Part model, mm, in its own coordinate system. A direction names the side the tool comes from. Give positions to 0.01 mm unless a question says otherwise; leave off trailing zeros. Write each loop counter-clockwise with the first axis right and the second up, starting at its lowest first coordinate (ties: lowest second). Pieces come first, ordered by that corner, then holes. Notation, with made-up numbers: M 28.25,-5 L 75.25,-5 A8 cw 75.25,10 Z; hole C 1,68 d8. An arc over 180 degrees is marked long. Answer as CSV lines item,"result". Start each with the question number.
Item 1: 3-axis set-ups, long thin cutter, end or side, ignore diameter. For faces 4 (the flat face through (-7, 1, 3.5)), 5 (the flat face through (0, 0, 16)), 6 (the flat face through (6, 1, 23.5)): which of +Z, -Z, +X, -X, +Y, -Y reach the whole face in a straight line?
Item 2: Band-saw the part on D-D, the plane y = -27. List the corners of the cut face in (x, z).
Item 3: Two-plate mould, pull along Z, no slides. Class faces 1 (the flat face through (0, 3, 16)), 2 (the cylindrical face through (0.301, -6.898, 45.386)), 3 (the flat face through (-5, 1, 6)): +Z half, -Z half, draft (parallel to the pull), parting line (faces both ways), or undercut.
Item 4: Pin check, flat tips, straight feed: pin 1 (1.5 mm diameter, centred on x = 7, y = 1, fed in from +Z); pin 2 (1.5 mm diameter, centred on x = 4.5, y = -30.5, fed in from -Z); pin 3 (1 mm diameter, centred on x = 3, y = -14, fed in from -Z). Stop position of each tip, or through.
Item 5: Wall check: L1, parallel to Y at x = 20.4, z = 10; L2, parallel to Y at x = 2.5, z = 4; L3, parallel to Y at x = 13, z = 38.5. Give the ranges that are in metal, low to high. Write a range as from..to.
Item 6: Band-saw the part on C-C, the plane y = -22. List the corners of the cut face in (x, z).
Item 7: Band-saw the part on B-B, the plane z = 26. List the corners of the cut face in (x, y).
Item 8: Band-saw the part on A-A, the plane x = -10.5. List the corners of the cut face in (y, z).
from build123d import *

# Parameters (mm, degrees)
SKETCH_2_W               = 43
SKETCH_2_H               = 32
EXTRUDE_1_DEPTH          = 3
EXTRUDE_2_DEPTH          = 43
SKETCH_4_W               = 3
SKETCH_4_H               = 5
CUT_EXTRUDE_1_DEPTH      = 67.543791262
SKETCH_5_R               = 0.4
CUT_EXTRUDE_2_DEPTH      = 3
CUT_EXTRUDE_START        = -40
SKETCH_5_3_R             = 0.4
CUT_EXTRUDE_3_DEPTH      = 3
CUT_EXTRUDE_4_DEPTH      = 77.255007413
CUT_EXTRUDE_4_DEPTH_BACK = 77.255007413
SKETCH_8_R               = 1.1
CUT_EXTRUDE_5_DEPTH      = 44.977948296


with BuildPart() as part:
    # 草图2 → 凸台-拉伸1 (new body)
    with BuildSketch(Plane(origin=(0, 0, 0), x_dir=(1, 0, 0), z_dir=(0, 1, 0))):
        with Locations((0, -16)):
            Rectangle(SKETCH_2_W, SKETCH_2_H)
    extrude(amount=EXTRUDE_1_DEPTH)

    # 草图3 → 凸台-拉伸2 (add)
    with BuildSketch(Plane(origin=(21.5, 0, 0), x_dir=(0, 0, -1), z_dir=(1, 0, 0))):
        with BuildLine():
            ThreePointArc((-37.829111907, -20.328529058), (-42.573878655, -7.967989086), (-32, 0))
            Line((-32, 0), (-23.339745962, 0))
            ThreePointArc((-23.339745962, 0), (-43.453167914, -2.948606038), (-39.418869699, -22.872673346))
            Line((-39.418869699, -22.872673346), (-7.193042045, -43.009605387))
            Line((-7.193042045, -43.009605387), (-5.603284253, -40.465461099))
            Line((-5.603284253, -40.465461099), (-37.829111907, -20.328529058))
        make_face()
    extrude(amount=-EXTRUDE_2_DEPTH)

    # 草图4 → 切除-拉伸1 (cut, through all)
    with BuildSketch(Plane.XZ):
        with Locations((6.5, 6)):
            Rectangle(SKETCH_4_W, SKETCH_4_H)
        with Locations((6.5, 21)):
            Rectangle(SKETCH_4_W, SKETCH_4_H)
        with Locations((-6.5, 6)):
            Rectangle(SKETCH_4_W, SKETCH_4_H)
        with Locations((-6.5, 21)):
            Rectangle(SKETCH_4_W, SKETCH_4_H)
    extrude(amount=-CUT_EXTRUDE_1_DEPTH, mode=Mode.SUBTRACT)

    # 草图5 → 切除-拉伸2 (cut)
    with BuildSketch(Plane(origin=(21.5, 0, 0), x_dir=(0, 0, -1), z_dir=(1, 0, 0))):
        with Locations((-10, 1.5)):
            Circle(SKETCH_5_R)
        with Locations((-44.015771199, -7.554533052)):
            Circle(SKETCH_5_R)
        with Locations((-23.359125072, -31.139147958)):
            Circle(SKETCH_5_R)
    extrude(amount=-CUT_EXTRUDE_2_DEPTH, mode=Mode.SUBTRACT)

    # 草图5<3> → 切除-拉伸3 (cut)
    with BuildSketch(Plane(origin=(21.5, 0, 0), x_dir=(0, 0, -1), z_dir=(1, 0, 0)).offset(CUT_EXTRUDE_START)):
        with Locations((-10, 1.5)):
            Circle(SKETCH_5_3_R)
        with Locations((-44.015771199, -7.554533052)):
            Circle(SKETCH_5_3_R)
        with Locations((-23.359125072, -31.139147958)):
            Circle(SKETCH_5_3_R)
    extrude(amount=-CUT_EXTRUDE_3_DEPTH, mode=Mode.SUBTRACT)

    # 草图6 → 切除-拉伸4 (cut, two sides: drawn at the far end of the back side and taken through both)
    with BuildSketch(Plane(origin=(21.5, 0, 0), x_dir=(0, 0, -1), z_dir=(1, 0, 0)).offset(-CUT_EXTRUDE_4_DEPTH_BACK)):
        Polygon((-18.06699493, -32.677270285), (-7.193042045, -43.009605387), (-5.603284253, -40.465461099), align=None)
    extrude(amount=CUT_EXTRUDE_4_DEPTH + CUT_EXTRUDE_4_DEPTH_BACK, mode=Mode.SUBTRACT)

    # 草图8 → 切除-拉伸5 (cut, through all)
    with BuildSketch(Plane(origin=(0, -26.194402521, 24.8896926), x_dir=(1, 0, 0), z_dir=(0, 0.7249301923221455, -0.6888223401282635))):
        with Locations(Location((16.5, 19.411523677, 0), (0, 0, 270))):
            Circle(SKETCH_8_R)
        with Locations(Location((16.5, 14.411523677, 0), (0, 0, 270))):
            Circle(SKETCH_8_R)
        with Locations(Location((0, 14.411523677, 0), (0, 0, 270))):
            Circle(SKETCH_8_R)
        with Locations(Location((0, 19.411523677, 0), (0, 0, 270))):
            Circle(SKETCH_8_R)
        with Locations(Location((-16.5, 19.411523677, 0), (0, 0, 270))):
            Circle(SKETCH_8_R)
        with Locations(Location((-16.5, 14.411523677, 0), (0, 0, 270))):
            Circle(SKETCH_8_R)
    extrude(amount=-CUT_EXTRUDE_5_DEPTH, mode=Mode.SUBTRACT)


solid = part.part
Output:
1,face 4,"+Y, -Y"
1,face 5,"-Z, +X, -X"
1,face 6,"+Y"
2,outline,"M -21.5,27.15 L 21.5,27.15 L 21.5,32.81 L -21.5,32.81 Z"
3,face 1,"draft"
3,face 2,"+Z half"
3,face 3,"undercut"
4,pin 1,"z = 40.33"
4,pin 2,"z = 20.35"
4,pin 3,"z = 42.43"
5,L1,"-41.26..-40.34, 0..1.1, 1.9..3"
5,L2,"0..3"
5,L3,"-23.45..-19.87, -2.13..1.4"
6,outline,"M -21.5,35.15 L 21.5,35.15 L 21.5,40.66 L -21.5,40.66 Z"
7,outline,"M -21.5,-31.26 L 21.5,-31.26 L 21.5,-27.72 L -21.5,-27.72 Z; M -21.5,0 L 21.5,0 L 21.5,3 L -21.5,3 Z"
8,outline,"M -43.01,7.19 L -32.68,18.07 L -20.33,37.83 A11 cw 0,32 L 0,0 L 3,0 L 3,32 A14 ccw -22.87,39.42 Z"
